Input: part model. Units: mm. Frame: model coordinates. Round coordinates to 2 decimals unless told otherwise and drop trailing zeros. Loops run counter-clockwise (first coordinate to the right, second up) from the corner with the lowest first, then second, coordinate; pieces in that order, holes last.
1) Section C-C, the plane x = 6. Return loops of the section in (y, z), and give its area (3 significant figures).
2) Section B-B, the plane y = 24. Return loops of the section in (x, z), and give its area (3 significant figures).
3) Section A-A, the plane z = 1.6. Return loops of the section in (x, y).
4) First-contact query: pin 1 (2.5 mm diameter, centred on x = 6, y = 24, fed in from +Z). Flat tip, straight axial feed; report the tip coordinate or a pass-through.
5) Ray query, line 1 along X through (y, z) = (24, 0.3); line 2 along X through (y, z) = (19.5, 1.2); line 3 along Y through (x, z) = (41.5, 0.3). Return the intervals inside material, ascending.
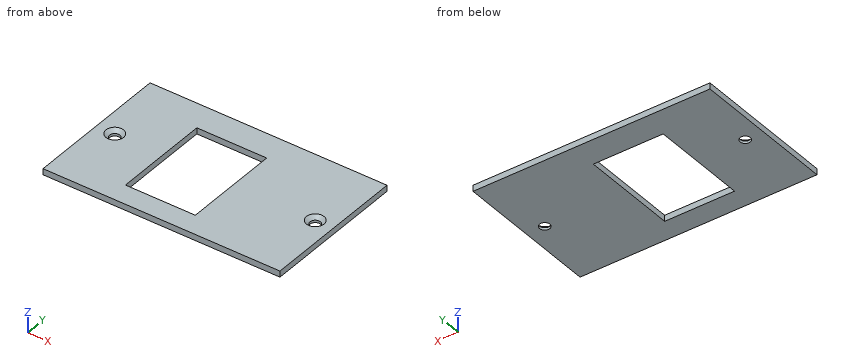
Autodesk Fusion 360 part; units mm, degrees
sketch "Sketch1" plane through (0, 0, 0) normal (0, 0, 1) x (1, 0, 0)
  line L0 (0, 0) -> (78, 0)
  line L1 (78, 0) -> (78, 48)
  line L2 (78, 48) -> (0, 48)
  line L3 (0, 48) -> (0, 0)
  dimension "d1" = 78
  dimension "d2" = 48
extrude "Extrude1" add sketch "Sketch1" along normal blind 2
sketch "Sketch2" plane through (0, 0, 2) normal (0, 0, 1) x (-1, 0, 0)
  line L0 (0, -48) -> (0, 0)
  line L1 (0, 0) -> (-78, 0)
  line L2 (-78, 0) -> (-78, -48)
  line L3 (-78, -48) -> (0, -48)
  point P0 (-72, -24)
  point P1 (-6, -24)
hole "Hole1" at (72, 24, 2) at (6, 24, 2) direction (0, 0, -1) diameter 3.4 depth 13 tip angle 118 countersink diameter 5.8 countersink angle 90
sketch "Sketch3" plane through (0, 0, 2) normal (0, 0, 1) x (-1, 0, 0)
  circle A0 centre (-72, -24) radius 2.9
  circle A1 centre (-6, -24) radius 2.9
  line L0 (0, -48) -> (0, 0)
  line L1 (0, 0) -> (-78, 0)
  line L2 (-78, 0) -> (-78, -48)
  line L3 (-78, -48) -> (0, -48)
  line L4 (-22, -39) -> (-45, -39)
  line L5 (-45, -39) -> (-45, -7)
  line L6 (-45, -7) -> (-22, -7)
  line L7 (-22, -7) -> (-22, -39)
extrude "Extrude2" cut sketch "Sketch3" against normal blind 500 contours L4 L5 L6 L7
Final values:
1. outline: (0, 0) - (22.3, 0) - (22.3, 0.8) - (21.1, 2) - (0, 2) - close; (25.7, 0) - (48, 0) - (48, 2) - (26.9, 2) - (25.7, 0.8) - close
1. area: 87.8 mm2
2. outline: (0, 0) - (4.3, 0) - (4.3, 0.8) - (3.1, 2) - (0, 2) - close; (7.7, 0) - (22, 0) - (22, 2) - (8.9, 2) - (7.7, 0.8) - close; (45, 0) - (70.3, 0) - (70.3, 0.8) - (69.1, 2) - (45, 2) - close; (73.7, 0) - (78, 0) - (78, 2) - (74.9, 2) - (73.7, 0.8) - close
2. area: 93.5 mm2
3. outline: (0, 0) - (78, 0) - (78, 48) - (0, 48) - close; hole circle Ø5 at (6, 24); hole (22, 7) - (45, 7) - (45, 39) - (22, 39) - close; hole circle Ø5 at (72, 24)
4. pin 1: passes through
5. line 1: x = 0 to 4.3, 7.7 to 22, 45 to 70.3, 73.7 to 78
5. line 2: x = 0 to 22, 45 to 78
5. line 3: y = 0 to 7, 39 to 48
